Input: part model. Units: mm. Frame: model coordinates. Round coordinates to 2 decimals unless told otherwise and drop trailing zeros. Order: outer loops, then holes, each group sorted by start corner. A loop starts at its lowest first (then second) coordinate and runs counter-clockwise, first axis right, second up.
Item 1: Cut plane C-C on x = 15. Output: boundary loops of the cut face in (y, z), then the cut area to 3 significant figures.
Item 2: First-contact query: pin 1 (3 mm diameter, centred on y = -1, z = -17.5, fed in from -X); pin 2 (2.5 mm diameter, centred on x = 16, z = -18.5, fed in from -Y). Flat tips, straight axial feed; report the tip coordinate or a pass-through.
Item 3: Cut plane A-A on z = -18.8. Give the number of separate pieces and of enclosed holes in the cut face, then the cut area to 3 significant figures.
Item 4: Cut plane D-D on y = -4. Output: boundary loops of the cut face in (x, z), then the cut area to 3 significant figures.
Item 5: Cut plane B-B on y = -26. Output: boundary loops of the cut face in (x, z), then the cut area to 3 significant figures.
Item 6: Line query: L1, parallel to X at y = 14, z = -17; L2, parallel to Y at x = 55, z = -19.4; L3, parallel to Y at x = 49, z = -19.5. Output: solid intervals per line, ascending.
```python
from build123d import *

# Parameters (mm, degrees)
BOX010_W          = 8
BOX010_H          = 9
BOX010_DEPTH      = 5
BOX011_W          = 8
BOX011_H          = 9
BOX011_DEPTH      = 5
CYLINDER012_R     = 2.5
CYLINDER012_DEPTH = 5
CYLINDER010_R     = 2.5
CYLINDER010_DEPTH = 5
CYLINDER009_R     = 2.5
CYLINDER009_DEPTH = 5
CYLINDER008_R     = 2.5
CYLINDER008_DEPTH = 5
CYLINDER005_R     = 2.5
CYLINDER005_DEPTH = 5
CYLINDER003_R     = 2.5
CYLINDER003_DEPTH = 5
CYLINDER004_R     = 2.5
CYLINDER004_DEPTH = 5
CYLINDER006_R     = 2.5
CYLINDER006_DEPTH = 5
CYLINDER007_R     = 2.5
CYLINDER007_DEPTH = 5
CYLINDER013_R     = 2.5
CYLINDER013_DEPTH = 5
BOX013_W          = 25
BOX013_H          = 26
BOX013_DEPTH      = 5
CYLINDER011_R     = 12.5
CYLINDER011_DEPTH = 5
BOX012_W          = 120
BOX012_H          = 16
BOX012_DEPTH      = 5


with BuildPart() as cube010:
    # Box010 → Box010 (new body)
    with BuildSketch(Plane(origin=(103, 8, 0), x_dir=(1, 0, 0), z_dir=(0, 0, 1))):
        with Locations((4, 4.5)):
            Rectangle(BOX010_W, BOX010_H)
    extrude(amount=BOX010_DEPTH)


with BuildPart() as cube011:
    # Box011 → Box011 (new body)
    with BuildSketch(Plane(origin=(-1, 8, 0), x_dir=(1, 0, 0), z_dir=(0, 0, 1))):
        with Locations((4, 4.5)):
            Rectangle(BOX011_W, BOX011_H)
    extrude(amount=BOX011_DEPTH)


with BuildPart() as zylinder012:
    # Cylinder012 → Cylinder012 (new body)
    with BuildSketch(Plane(origin=(6, -6, 0), x_dir=(1, 0, 0), z_dir=(0, 0, 1))):
        Circle(CYLINDER012_R)
    extrude(amount=CYLINDER012_DEPTH)


with BuildPart() as zylinder010:
    # Cylinder010 → Cylinder010 (new body)
    with BuildSketch(Plane(origin=(-6, -6, 0), x_dir=(1, 0, 0), z_dir=(0, 0, 1))):
        Circle(CYLINDER010_R)
    extrude(amount=CYLINDER010_DEPTH)


with BuildPart() as zylinder009:
    # Cylinder009 → Cylinder009 (new body)
    with BuildSketch(Plane(origin=(0, -6, 0), x_dir=(1, 0, 0), z_dir=(0, 0, 1))):
        Circle(CYLINDER009_R)
    extrude(amount=CYLINDER009_DEPTH)


with BuildPart() as zylinder008:
    # Cylinder008 → Cylinder008 (new body)
    with BuildSketch(Plane(origin=(0, 6, 0), x_dir=(1, 0, 0), z_dir=(0, 0, 1))):
        Circle(CYLINDER008_R)
    extrude(amount=CYLINDER008_DEPTH)


with BuildPart() as zylinder005:
    # Cylinder005 → Cylinder005 (new body)
    with BuildSketch(Plane(origin=(-3, 0, 0), x_dir=(1, 0, 0), z_dir=(0, 0, 1))):
        Circle(CYLINDER005_R)
    extrude(amount=CYLINDER005_DEPTH)


with BuildPart() as zylinder003:
    # Cylinder003 → Cylinder003 (new body)
    with BuildSketch(Plane(origin=(3, 0, 0), x_dir=(1, 0, 0), z_dir=(0, 0, 1))):
        Circle(CYLINDER003_R)
    extrude(amount=CYLINDER003_DEPTH)


with BuildPart() as zylinder004:
    # Cylinder004 → Cylinder004 (new body)
    with BuildSketch(Plane(origin=(9, 0, 0), x_dir=(1, 0, 0), z_dir=(0, 0, 1))):
        Circle(CYLINDER004_R)
    extrude(amount=CYLINDER004_DEPTH)


with BuildPart() as zylinder006:
    # Cylinder006 → Cylinder006 (new body)
    with BuildSketch(Plane(origin=(-9, 0, 0), x_dir=(1, 0, 0), z_dir=(0, 0, 1))):
        Circle(CYLINDER006_R)
    extrude(amount=CYLINDER006_DEPTH)


with BuildPart() as zylinder007:
    # Cylinder007 → Cylinder007 (new body)
    with BuildSketch(Plane(origin=(-6, 6, 0), x_dir=(1, 0, 0), z_dir=(0, 0, 1))):
        Circle(CYLINDER007_R)
    extrude(amount=CYLINDER007_DEPTH)


with BuildPart() as fusion007:
    # Cylinder013 → Cylinder013 (new body)
    with BuildSketch(Plane(origin=(6, 6, 0), x_dir=(1, 0, 0), z_dir=(0, 0, 1))):
        Circle(CYLINDER013_R)
    extrude(amount=CYLINDER013_DEPTH)

    # Fusion005: union Zylinder012, Zylinder010, Zylinder009, Zylinder008, Zylinder005, Zylinder003, Zylinder004, Zylinder006, Zylinder007
    add(zylinder012.part)
    add(zylinder010.part)
    add(zylinder009.part)
    add(zylinder008.part)
    add(zylinder005.part)
    add(zylinder003.part)
    add(zylinder004.part)
    add(zylinder006.part)
    add(zylinder007.part)


with BuildPart() as fusion007_1:
    # Fusion005 placement: moved
    add(fusion007.part.moved(Location((55, -20, 0))))

    # Fusion007: union Cube010, Cube011
    add(cube010.part)
    add(cube011.part)


with BuildPart() as cube013:
    # Box013 → Box013 (new body)
    with BuildSketch(Plane(origin=(42.5, -20, 0), x_dir=(1, 0, 0), z_dir=(0, 0, 1))):
        with Locations((12.5, 13)):
            Rectangle(BOX013_W, BOX013_H)
    extrude(amount=BOX013_DEPTH)


with BuildPart() as zylinder011:
    # Cylinder011 → Cylinder011 (new body)
    with BuildSketch(Plane(origin=(55, -20, 0), x_dir=(1, 0, 0), z_dir=(0, 0, 1))):
        Circle(CYLINDER011_R)
    extrude(amount=CYLINDER011_DEPTH)


with BuildPart() as obj1:
    # Box012 → Box012 (new body)
    with BuildSketch(Plane(origin=(-5, 4, 0), x_dir=(1, 0, 0), z_dir=(0, 0, 1))):
        with Locations((60, 8)):
            Rectangle(BOX012_W, BOX012_H)
    extrude(amount=BOX012_DEPTH)

    # Fusion006: union Cube013, Zylinder011
    add(cube013.part)
    add(zylinder011.part)

    # Cut003: cut Fusion007
    add(fusion007_1.part, mode=Mode.SUBTRACT)


with BuildPart() as obj1_1:
    # Cut003 placement: moved
    add(obj1.part.moved(Location((0, 0, -21))))


solid = obj1_1.part
```
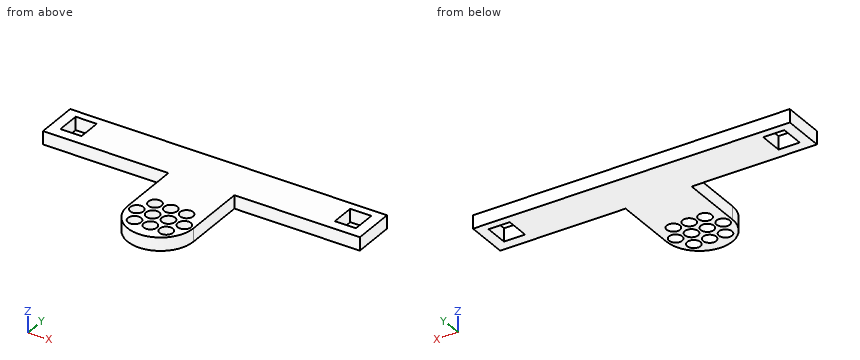
From the geometry:
1. outline: (4, -21) - (20, -21) - (20, -16) - (4, -16) - close
1. area: 80.0 mm2
2. pin 1: stops at x = 42.5
2. pin 2: stops at y = 4
3. separate pieces: 1
3. enclosed holes: 12
3. area: 2,430 mm2
4. outline: (42.5, -21) - (67.5, -21) - (67.5, -16) - (42.5, -16) - close
4. area: 125 mm2
5. outline: (44.03, -21) - (46.5, -21) - (46.5, -16) - (44.03, -16) - close; (51.5, -21) - (52.5, -21) - (52.5, -16) - (51.5, -16) - close; (57.5, -21) - (58.5, -21) - (58.5, -16) - (57.5, -16) - close; (63.5, -21) - (65.97, -21) - (65.97, -16) - (63.5, -16) - close
5. area: 34.7 mm2
6. L1: x = -5 to -1, 7 to 103, 111 to 115
6. L2: y = -32.5 to -28.5, -23.5 to -16.5, -11.5 to 20
6. L3: y = -30.97 to -28.5, -23.5 to -16.5, -11.5 to 20
